Model file for the job. Use its own axes, mm. A direction names the side the tool comes from. Round coordinates to 2 decimals unless told otherwise and drop trailing zeros. Order: outer loops, then holes, each group sorted by start corner. A loop starts at its lowest first (then second) coordinate and runs counter-clockwise, first axis right, second up. Notation, with made-up numbers: (23.25, 37) - (56.25, 37) arc R25 ccw to (56.25, 55) - close; hole circle Ø1 at (54, -27). An arc over 180 degrees is marked (long way). Use one line per item in the form item = value.
from build123d import *

# Parameters (mm, degrees)
EXTRUDE_1_DEPTH = 200
EXTRUDE_2_DEPTH = 10
EXTRUDE_3_DEPTH = 10
FILLET_1_R      = 10
EXTRUDE_4_REACH = 206.695
SKETCH_4_R      = 2.5
SKETCH_5_R      = 5
EXTRUDE_5_DEPTH = 30
EXTRUDE_6_DEPTH = 10


with BuildPart() as part:
    # 스케치1 → 보스-돌출1 (new body)
    with BuildSketch(Plane(origin=(0, 0, 0), x_dir=(0, 0, -1), z_dir=(1, 0, 0))):
        Polygon((30, 0), (-30, 0), (-30, 20), (-10, 20), (-10, 40), (10, 40), (10, 20), (30, 20), align=None)
    extrude(amount=EXTRUDE_1_DEPTH)

    # 스케치2 → 보스-돌출2 (add)
    with BuildSketch(Plane.ZY):
        Polygon((-30, 20), (-20, 20), (-20, 60), (20, 60), (20, 20), (30, 20), (30, 70), (-30, 70), align=None)
    extrude(amount=-EXTRUDE_2_DEPTH)

    # 스케치3 → 보스-돌출3 (add)
    with BuildSketch(Plane.ZY.offset(-100)):
        Polygon((20, 20), (30, 20), (30, 70), (-30, 70), (-30, 20), (-20, 20), (-20, 60), (20, 60), align=None)
    extrude(amount=-EXTRUDE_3_DEPTH)

    # 필렛1
    fillet_1_edges = [part.edges().sort_by_distance(p)[0] for p in [
        (5, 70, -30),
        (5, 70, 30),
        (105, 70, -30),
        (105, 70, 30),
    ]]
    fillet(fillet_1_edges, radius=FILLET_1_R)

    # 스케치4 → 보스-돌출4 (add, up to next)
    with BuildSketch(Plane(origin=(10, 0, 0), x_dir=(0, 0, -1), z_dir=(1, 0, 0)), mode=Mode.PRIVATE) as extrude_4_sk1:
        with Locations((0, 65)):
            Circle(SKETCH_4_R)
    extrude_4_tool1 = extrude(extrude_4_sk1.sketch, amount=EXTRUDE_4_REACH, mode=Mode.PRIVATE) - part.part
    add(extrude_4_tool1.solids().sort_by_distance((10, 65, 0))[0])

    # 스케치5 → 보스-돌출5 (add)
    with BuildSketch(Plane(origin=(0, 40, 0), x_dir=(1, 0, 0), z_dir=(0, 1, 0))):
        with Locations(Location((160, 0, 0), (0, 0, 90))):
            Circle(SKETCH_5_R)
    extrude(amount=EXTRUDE_5_DEPTH)

    # 스케치6 → 보스-돌출6 (add)
    with BuildSketch(Plane.ZY):
        with BuildLine():
            Line((-1.5, 73), (-1.5, 70))
            Line((-1.5, 70), (1.5, 70))
            Line((1.5, 70), (1.5, 73))
            ThreePointArc((1.5, 73), (0, 71.5), (-1.5, 73))
        make_face()
    extrude(amount=-EXTRUDE_6_DEPTH)


solid = part.part
(1) Slice it at C-C on x = 102. Give the cut face in (y, z).
Report:
outline = (0, -30) - (60, -30) arc R10 ccw to (70, -20) - (70, 20) arc R10 ccw to (60, 30) - (0, 30) - close; hole (20, -20) - (60, -20) - (60, 20) - (20, 20) - (20, 10) - (40, 10) - (40, -10) - (20, -10) - close
(2) Slice it at A-A on x = 28.5. Give the cut face in (y, z), then the cut area to 3 significant figures.
Report:
outline = (0, -30) - (20, -30) - (20, -10) - (40, -10) - (40, 10) - (20, 10) - (20, 30) - (0, 30) - close; circle Ø5 at (65, 0)
area = 1,620 mm2
(3) Slice it at B-B on y = 44. Give the cut face in (x, z), then the cut area to 3 significant figures.
Report:
outline = (0, -30) - (10, -30) - (10, -20) - (0, -20) - close; (0, 20) - (10, 20) - (10, 30) - (0, 30) - close; (100, -30) - (110, -30) - (110, -20) - (100, -20) - close; (100, 20) - (110, 20) - (110, 30) - (100, 30) - close; circle Ø10 at (160, 0)
area = 479 mm2
(4) Probe probe 1 along X at (y, z) = (23, 26.5); probe 2 along Z at (x, y) = (101, 25.5); probe 3 along Y at (x, z) = (79, -3). List the from-to ranges inside material, lowest first. Write a range as [from, to].
Report:
probe_1 = [0, 10], [100, 110]
probe_2 = [-30, -20], [-10, 10], [20, 30]
probe_3 = [0, 40]
(5) Slice it at D-D on z = -12.5. Give the cut face in (x, y), then the cut area to 3 significant figures.
Report:
outline = (0, 0) - (200, 0) - (200, 20) - (0, 20) - close; (0, 60) - (10, 60) - (10, 70) - (0, 70) - close; (100, 60) - (110, 60) - (110, 70) - (100, 70) - close
area = 4,200 mm2
(6) Pin check, flat tips, straight feed: pin 1 (5 mm diameter, centred on x = 35, z = 9, fed in from +Y); pin 2 (8 mm diameter, centred on x = 90, y = 28.5, fed in from -Z); pin 3 (10 mm diameter, centred on x = 72.5, z = 18, fed in from +Y). Stop position of each tip, or through.
Report:
pin_1 = 40
pin_2 = -10
pin_3 = 20
(7) Tool access for faces 5 (the face through (105, 40, 20)), 6 (the face through (5, 70, 11)), 7 (the face through (5, 60, 0)): list every direction of +Z, -Z, +X, -X, +Y, -Y with a clear straight run to the whole face (end or side of a thin tool).
Report:
face_5 = +X, -X
face_6 = +Z, +X, -X, +Y
face_7 = -X
(8) Pull direction X, two halves, no side cores. Call faces 1 (the face through (10, 46.9, -20.4)), 2 (the face through (99, 20, 20)), 3 (the face through (200, 16, 0)), 4 (the face through (99, 30, -10)): released by +X, released by -X, zero draft, split by the parting line, or undercut.
Report:
face_1 = undercut
face_2 = undercut
face_3 = released by +X
face_4 = zero draft
